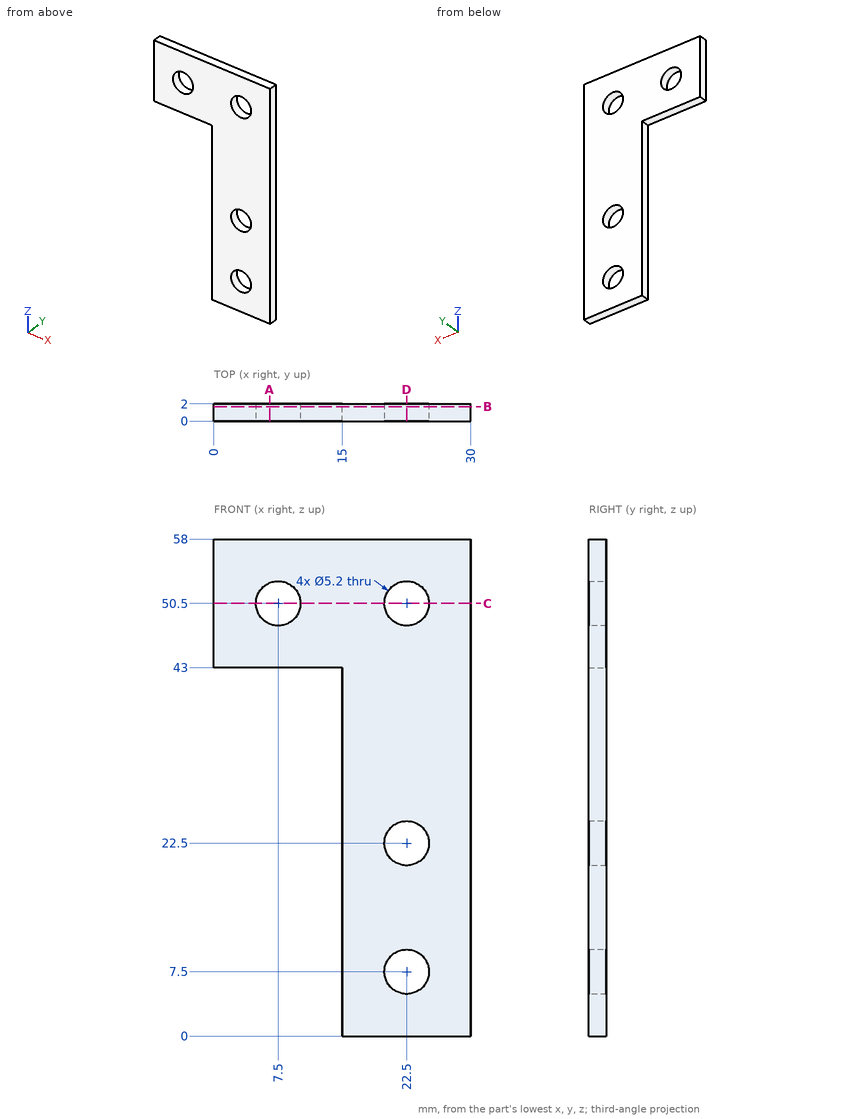
Verification items for this drawing (mm, ordinates from the low corner). Coordinates: 2 decimals unless noted, no trailing zeros. Loops run counter-clockwise (first coordinate to the right, second up) from the corner with the lowest first, then second, coordinate; pieces in that order, holes last. Notation, with made-up numbers: (42, 55.5) -> (97, 55.5) arc R35 ccw to (97, 94.5) -> close; hole circle Ø2 at (33.25, 47.5). An arc over 180 degrees is marked (long way). Answer in a Markdown table with one row per item. Add a question column.
1. Section check C-C, the plane z = 50.5. Enter the section's corners in (x, y).
2. Material ranges on probe 1 along X at (y, z) = (0.7, 50.5); probe 2 along Z at (x, y) = (24.5, 0.7); probe 3 along Z at (x, y) = (24, 1), recorded low to high. Write a range as [from, to].
3. Section check A-A, the plane x = 6.5. Enter the section's corners in (y, z).
4. Section check D-D, the plane x = 22.5. Enter the section's corners in (y, z).
5. Section check B-B, the plane y = 1.7. Enter the section's corners in (x, z), then the cut area to 3 significant figures.
6. Depth check by flat-ended pin: P1, Ø3, axis at x = 22.5, z = 22.5, coming from the -Y side; P2, Ø0.6, axis at x = 7.5, y = 1, coming from the -Z side. Enter the tip coordinate at first touch or a pass-through.
Derived:
| question | item | result |
|---|---|---|
| 1 | outline | (0, 0) -> (4.9, 0) -> (4.9, 2) -> (0, 2) -> close; (10.1, 0) -> (19.9, 0) -> (19.9, 2) -> (10.1, 2) -> close; (25.1, 0) -> (30, 0) -> (30, 2) -> (25.1, 2) -> close |
| 2 | probe 1 | x = [0, 4.9], [10.1, 19.9], [25.1, 30] |
| 2 | probe 2 | z = [0, 5.84], [9.16, 20.84], [24.16, 48.84], [52.16, 58] |
| 2 | probe 3 | z = [0, 5.38], [9.62, 20.38], [24.62, 48.38], [52.62, 58] |
| 3 | outline | (0, 43) -> (2, 43) -> (2, 48.1) -> (0, 48.1) -> close; (0, 52.9) -> (2, 52.9) -> (2, 58) -> (0, 58) -> close |
| 4 | outline | (0, 0) -> (2, 0) -> (2, 4.9) -> (0, 4.9) -> close; (0, 10.1) -> (2, 10.1) -> (2, 19.9) -> (0, 19.9) -> close; (0, 25.1) -> (2, 25.1) -> (2, 47.9) -> (0, 47.9) -> close; (0, 53.1) -> (2, 53.1) -> (2, 58) -> (0, 58) -> close |
| 5 | outline | (0, 43) -> (15, 43) -> (15, 0) -> (30, 0) -> (30, 58) -> (0, 58) -> close; hole circle Ø5.2 at (7.5, 50.5); hole circle Ø5.2 at (22.5, 7.5); hole circle Ø5.2 at (22.5, 22.5); hole circle Ø5.2 at (22.5, 50.5) |
| 5 | area | 1,010 mm² |
| 6 | P1 | passes through |
| 6 | P2 | stops at z = 43 |
